from build123d import *
from build123d.topology import SkipClean

# Parameters (mm, degrees)
SKETCH1_W              = 39.5
SKETCH1_H              = 29
BOSS_EXTRUDE1_DEPTH    = 2
SKETCH2_R              = 13.5
SKETCH2_R_2            = 8.5
BOSS_EXTRUDE2_DEPTH    = 10
SKETCH3_R              = 12.5
CUT_EXTRUDE1_DEPTH     = 2
SKETCH4_R              = 7.5
CUT_EXTRUDE2_DEPTH     = 9
CUT_EXTRUDE3_START     = -10.3
CUT_EXTRUDE3_DEPTH     = 20.6
BOSS_EXTRUDE3_DEPTH    = 10
SKETCH10_W             = 39.5
SKETCH10_H             = 29
SKETCH10_R             = 13.5
CUT_EXTRUDE4_DEPTH     = 10
SKETCH11_R             = 13.5
SKETCH11_W             = 14
SKETCH11_H             = 20.6
BOSS_EXTRUDE4_DEPTH    = 8
SKETCH12_R             = 13.5
SKETCH12_R_2           = 12.5
BOSS_EXTRUDE5_DEPTH    = 2
CUT_SWEEP2_START       = -214.83981443
CUT_SWEEP2_OUTLINE_R   = 0.6
CUT_SWEEP2_DEPTH       = 22.83981443
CUT_SWEEP2_2_OUTLINE_R = 0.6
CUT_SWEEP2_2_ANGLE     = 17.195102
CUT_SWEEP2_START_2     = -205
CUT_SWEEP2_3_OUTLINE_R = 0.6
CUT_SWEEP2_3_DEPTH     = 2.526605635
BOSS_EXTRUDE7_DEPTH    = 10.25
CUT_EXTRUDE5_DEPTH     = 8
SKETCH20_R             = 1.6
CUT_EXTRUDE6_DEPTH     = 4
SKETCH21_R             = 2.5
SKETCH21_R_2           = 1.6
BOSS_EXTRUDE8_DEPTH    = 4
SKETCH22_W             = 4
SKETCH22_H             = 4
BOSS_EXTRUDE9_DEPTH    = 27
BOSS_EXTRUDE11_DEPTH   = 10
SKETCH8_2_R            = 0.6
SKETCH24_R             = 1.1
CUT_EXTRUDE7_DEPTH     = 1.1


with BuildPart() as part:
    # Sketch1 → Boss-Extrude1 (new body)
    with BuildSketch(Plane(origin=(0, 0, 0), x_dir=(1, 0, 0), z_dir=(0, 1, 0))):
        with Locations((-212.126239175, -24.349172792)):
            Rectangle(SKETCH1_W, SKETCH1_H)
    extrude(amount=BOSS_EXTRUDE1_DEPTH)

    # Sketch2 → Boss-Extrude2 (add)
    with BuildSketch(Plane(origin=(0, 2, 0), x_dir=(1, 0, 0), z_dir=(0, 1, 0))):
        with Locations((-206.876239175, -24.349172792)):
            Circle(SKETCH2_R)
        with Locations((-222.376239175, -24.349172792)):
            Circle(SKETCH2_R_2)
    extrude(amount=BOSS_EXTRUDE2_DEPTH)

    # Sketch3 → Cut-Extrude1 (cut)
    with BuildSketch(Plane(origin=(0, 12, 0), x_dir=(1, 0, 0), z_dir=(0, 1, 0))):
        with Locations(Location((-206.876239175, -24.349172792, 0), (0, 0, 270))):
            Circle(SKETCH3_R)
    extrude(amount=-CUT_EXTRUDE1_DEPTH, mode=Mode.SUBTRACT)

    # Sketch4 → Cut-Extrude2 (cut)
    with BuildSketch(Plane(origin=(0, 12, 0), x_dir=(1, 0, 0), z_dir=(0, 1, 0))):
        with Locations(Location((-222.376239175, -24.349172792, 0), (0, 0, 270))):
            Circle(SKETCH4_R)
    extrude(amount=-CUT_EXTRUDE2_DEPTH, mode=Mode.SUBTRACT)

    # Cut-Extrude3: read off the stored shape, not the designer's step
    # Cut-Extrude3 outline → Cut-Extrude3 (cut)
    with BuildSketch(Plane.XY.offset(24.349172792).offset(CUT_EXTRUDE3_START)):
        with BuildLine():
            ThreePointArc((-213.876239175, 8), (-206.876239175, 1), (-199.876239175, 8))
            Line((-199.876239175, 8), (-199.876239175, 10))
            Line((-199.876239175, 10), (-213.876239175, 10))
            Line((-213.876239175, 10), (-213.876239175, 8))
        make_face()
    extrude(amount=CUT_EXTRUDE3_DEPTH, mode=Mode.SUBTRACT)

    # Sketch7 → Boss-Extrude3 (add)
    with BuildSketch(Plane(origin=(0, 2, 0), x_dir=(1, 0, 0), z_dir=(0, 1, 0))):
        with BuildLine():
            Line((-192.376239175, -26.349172792), (-192.376239175, -24.349172792))
            Line((-192.376239175, -24.349172792), (-192.376239175, -22.349172792))
            Line((-192.376239175, -22.349172792), (-193.525209252, -22.349172792))
            ThreePointArc((-193.525209252, -22.349172792), (-193.413533207, -23.346402619), (-193.376239175, -24.349172792))
            ThreePointArc((-193.376239175, -24.349172792), (-193.413533207, -25.351942966), (-193.525209252, -26.349172792))
            Line((-193.525209252, -26.349172792), (-192.376239175, -26.349172792))
        make_face()
    extrude(amount=BOSS_EXTRUDE3_DEPTH)

    # Sketch10 → Cut-Extrude4 (cut)
    with BuildSketch(Plane(origin=(0, 2, 0), x_dir=(1, 0, 0), z_dir=(0, 1, 0))):
        with Locations((-212.126239175, -24.349172792)):
            Rectangle(SKETCH10_W, SKETCH10_H)
        with Locations(Location((-206.876239175, -24.349172792, 0), (0, 0, 151.062655238))):
            Circle(SKETCH10_R, mode=Mode.SUBTRACT)
    extrude(amount=CUT_EXTRUDE4_DEPTH, mode=Mode.SUBTRACT)

    # Sketch11 → Boss-Extrude4 (add)
    with BuildSketch(Plane(origin=(0, 2, 0), x_dir=(1, 0, 0), z_dir=(0, 1, 0))):
        with Locations(Location((-206.876239175, -24.349172792, 0), (0, 0, 151.062655238))):
            Circle(SKETCH11_R)
        with Locations((-206.876239175, -24.349172792)):
            Rectangle(SKETCH11_W, SKETCH11_H, mode=Mode.SUBTRACT)
    extrude(amount=BOSS_EXTRUDE4_DEPTH)

    # Sketch12 → Boss-Extrude5 (add)
    with SkipClean():  # the faces are left unmerged after this step: merging them gives an invalid solid
        with BuildSketch(Plane(origin=(0, 10, 0), x_dir=(1, 0, 0), z_dir=(0, 1, 0))):
            with Locations(Location((-206.876239175, -24.349172792, 0), (0, 0, 270))):
                Circle(SKETCH12_R)
            with Locations(Location((-206.876239175, -24.349172792, 0), (0, 0, 270))):
                Circle(SKETCH12_R_2, mode=Mode.SUBTRACT)
        extrude(amount=BOSS_EXTRUDE5_DEPTH)
    add(part.part.scale(1), mode=Mode.REPLACE)  # the faces are merged on a copy

    # Cut-Sweep2: read off the stored shape, not the designer's step
    # Cut-Sweep2 outline → Cut-Sweep2 (cut)
    with SkipClean():  # the faces are left unmerged after this step: merging them gives an invalid solid
        with BuildSketch(Plane.YZ.offset(CUT_SWEEP2_START)):
            with Locations((8.75, 24.349172792)):
                Circle(CUT_SWEEP2_OUTLINE_R)
        extrude(amount=CUT_SWEEP2_DEPTH, mode=Mode.SUBTRACT)

    # Cut-Sweep2 2 outline → Cut-Sweep2 2 (revolve, cut)
    with SkipClean():  # the faces are left unmerged after this step: merging them gives an invalid solid
        with BuildSketch(Plane(origin=(-214.83981433, 0, 9.349172792), x_dir=(-0.2956263792524328, 0, 0.9553036396298806), z_dir=(-0.9553036396298806, 0, -0.2956263792524328))):
            with Locations((15, 8.75)):
                Circle(CUT_SWEEP2_2_OUTLINE_R)
        revolve(axis=Axis((-214.83981433, 0, 9.349172792), (0, 1, 0)), revolution_arc=CUT_SWEEP2_2_ANGLE, mode=Mode.SUBTRACT)

    # Cut-Sweep2 3 outline → Cut-Sweep2 3 (cut)
    with SkipClean():  # the faces are left unmerged after this step: merging them gives an invalid solid
        with BuildSketch(Plane(origin=(0, 0, 0), x_dir=(0, 1, 0), z_dir=(0.9553036396298961, 0, 0.29562637925238305)).offset(CUT_SWEEP2_START_2)):
            with Locations((8.75, 87.443615225)):
                Circle(CUT_SWEEP2_3_OUTLINE_R)
        extrude(amount=CUT_SWEEP2_3_DEPTH, mode=Mode.SUBTRACT)

    # Sketch18 → Boss-Extrude7 (add)
    with SkipClean():  # the faces are left unmerged after this step: merging them gives an invalid solid
        with BuildSketch(Plane(origin=(0, 2, 0), x_dir=(1, 0, 0), z_dir=(0, 1, 0))):
            Polygon((-228.567210955, -11.746276031), (-229.459691419, -19.696337579), (-226.478418338, -20.031017753), (-225.585937874, -12.080956204), align=None)
            Polygon((-225.585937874, -12.080956204), (-226.478418338, -20.031017753), (-223.497145257, -20.365697927), (-222.604664794, -12.415636378), align=None)
            Polygon((-227.482458859, -28.974836995), (-226.92465857, -24.006048527), (-229.90593165, -23.671368353), (-230.46373194, -28.640156821), align=None)
            Polygon((-223.943385489, -24.340728701), (-226.92465857, -24.006048527), (-227.482458859, -28.974836995), (-224.501185779, -29.309517169), align=None)
        extrude(amount=BOSS_EXTRUDE7_DEPTH)

    # Sketch19 → Cut-Extrude5 (cut)
    with SkipClean():  # the faces are left unmerged after this step: merging them gives an invalid solid
        with BuildSketch(Plane(origin=(-5.039382401, 0, 44.889946486), x_dir=(0.9937576935397466, 0, 0.11156005795338761), z_dir=(-0.11156005795338761, 0, 0.9937576935397466))):
            Polygon((-222.830009143, 12.25), (-224.430009143, 12.25), (-224.430009143, 10.65), (-221.230009143, 10.65), (-221.230009143, 12.25), align=None)
        extrude(amount=-CUT_EXTRUDE5_DEPTH, mode=Mode.SUBTRACT)

    # Sketch20 → Cut-Extrude6 (cut)
    with SkipClean():  # the faces are left unmerged after this step: merging them gives an invalid solid
        with BuildSketch(Plane(origin=(-5.485622633, 0, 48.864977261), x_dir=(-0.9937576935397466, 0, -0.11156005795338761), z_dir=(0.11156005795338761, 0, -0.9937576935397466))):
            with Locations((222.830009143, 12.25)):
                Circle(SKETCH20_R)
        extrude(amount=-CUT_EXTRUDE6_DEPTH, mode=Mode.SUBTRACT)

    # Sketch21 → Boss-Extrude8 (add)
    with SkipClean():  # the faces are left unmerged after this step: merging them gives an invalid solid
        with BuildSketch(Plane(origin=(-5.485622633, 0, 48.864977261), x_dir=(-0.9937576935397466, 0, -0.11156005795338761), z_dir=(0.11156005795338761, 0, -0.9937576935397466))):
            with Locations((222.830009143, 12.25)):
                Circle(SKETCH21_R)
            with Locations((222.830009143, 12.25)):
                Circle(SKETCH21_R_2, mode=Mode.SUBTRACT)
        extrude(amount=-BOSS_EXTRUDE8_DEPTH)

    # Sketch22 → Boss-Extrude9 (add)
    with SkipClean():  # the faces are left unmerged after this step: merging them gives an invalid solid
        with BuildSketch(Plane(origin=(0, 2, 0), x_dir=(1, 0, 0), z_dir=(0, 1, 0))):
            with Locations((-229.876239175, -11.849172792)):
                Rectangle(SKETCH22_W, SKETCH22_H)
            with Locations((-229.876239175, -36.849172792)):
                Rectangle(SKETCH22_W, SKETCH22_H)
            with Locations((-194.376239175, -36.849172792)):
                Rectangle(SKETCH22_W, SKETCH22_H)
            with Locations((-194.376239175, -11.849172792)):
                Rectangle(SKETCH22_W, SKETCH22_H)
        extrude(amount=BOSS_EXTRUDE9_DEPTH)

    # Sketch23 → Boss-Extrude11 (add)
    with BuildSketch(Plane(origin=(0, 2, 0), x_dir=(1, 0, 0), z_dir=(0, 1, 0))):
        with BuildLine():
            Line((-193.376239175, -24.349172792), (-192.376239175, -24.349172792))
            Line((-192.376239175, -24.349172792), (-192.376239175, -22.349172792))
            Line((-192.376239175, -22.349172792), (-193.525209252, -22.349172792))
            ThreePointArc((-193.525209252, -22.349172792), (-193.413533207, -23.346402619), (-193.376239175, -24.349172792))
        make_face()
        with BuildLine():
            Line((-192.376239175, -26.349172792), (-192.376239175, -24.349172792))
            Line((-192.376239175, -24.349172792), (-193.376239175, -24.349172792))
            ThreePointArc((-193.376239175, -24.349172792), (-193.413533207, -25.351942966), (-193.525209252, -26.349172792))
            Line((-193.525209252, -26.349172792), (-192.376239175, -26.349172792))
        make_face()
    extrude(amount=BOSS_EXTRUDE11_DEPTH)

    # Cut-Sweep3: sweep along a path in Sketch17<2>
    with SkipClean():  # the faces are left unmerged after this step: merging them gives an invalid solid
        with BuildLine(Plane(origin=(0, 8.75, 0), x_dir=(1, 0, 0), z_dir=(0, 1, 0))) as cut_sweep3_path:
            Line((-192.376239175, -24.349172792), (-213.876239175, -24.349172792))
            Line((-213.876239175, -24.349172792), (-214.83981433, -24.349172792))
            ThreePointArc((-214.83981433, -24.349172792), (-217.08221049, -24.180614376), (-219.274210018, -23.678727387))
            Line((-219.274210018, -23.678727387), (-220.339151193, -23.349172792))
        # Sketch8<2> → Cut-Sweep3 (sweep, cut)
        with BuildSketch(Plane(origin=(-192.376239175, 0, 0), x_dir=(0, 0, -1), z_dir=(1, 0, 0))):
            with Locations((-24.349172792, 8.75)):
                Circle(SKETCH8_2_R)
        sweep(path=cut_sweep3_path.line, mode=Mode.SUBTRACT)
    add(part.part.scale(1), mode=Mode.REPLACE)  # the faces are merged on a copy

    # Sketch24 → Cut-Extrude7 (cut)
    with BuildSketch(Plane(origin=(0, 29, 0), x_dir=(1, 0, 0), z_dir=(0, 1, 0))):
        with Locations(Location((-229.876239175, -11.849172792, 0), (0, 0, 270))):
            Circle(SKETCH24_R)
        with Locations(Location((-229.876239175, -36.849172792, 0), (0, 0, 270))):
            Circle(SKETCH24_R)
        with Locations(Location((-194.376239175, -36.849172792, 0), (0, 0, 270))):
            Circle(SKETCH24_R)
        with Locations(Location((-194.376239175, -11.849172792, 0), (0, 0, 270))):
            Circle(SKETCH24_R)
    extrude(amount=-CUT_EXTRUDE7_DEPTH, mode=Mode.SUBTRACT)


solid = part.part
Build history of the part. All positions in model axes, mm. A direction names the side the tool comes from. Round coordinates to 2 decimals unless told otherwise and drop trailing zeros. Write each loop counter-clockwise with the first axis right and the second up, starting at its lowest first coordinate (ties: lowest second). Pieces come first, ordered by that corner, then holes. Notation, with made-up numbers: M -35,15.25 L -26,15.25 A20 ccw -26,30.25 Z; hole C 25.25,84 d6. An arc over 180 degrees is marked long. Answer as a JSON object with one key per item and string values. Group by question number.
(1) Cut at A-A (y = 19.5). Give the cut face in (x, z).
(2) Flat gauge pins, fed straight in: pin 1 (2.5 mm diameter, centred on x = -194.5, z = 37, fed in from +Y); pin 2 (0.7 mm diameter, centred on x = -223.5, z = 15.5, fed in from +Y); pin 3 (3 mm diameter, centred on y = 9.5, z = 19, fed in from +X); pin 4 (1 mm diameter, centred on y = 8.5, z = 20, fed in from -X). Where does each tip first touch, or does it go through?
(3) Cut at B-B (x = -208.5). Give the cut face in (y, z).
(4) Which spindle directions (+Z, -Z, +X, -X, +Y, -Y) get a long thin tool onto all of the face, cutting with end or side? Do faces 1 (the flat face through (-224.45, 11.44, 16.29)), 2 (the flat face through (-230, 15, 34.849)), 3 (the flat face through (-194, 15, 13.849)), 4 (the flat face through (-207, 7, 14.049)), 5 (the flat face through (-224.226, 7.053, 26.86)). Say none if no direction does.
(5) Cut at C-C (z = 19). Give the cut face in (x, y).
(6) Cut at D-D (y = 2.5). Give the number of separate pieces and of enclosed holes in the cut face, and give its area (3 significant figures).
(7) Mould opens along X. For faces 6 (the flat face through (-212, 0, 24)), 7 (the flat face through (-196.376, 15, 37)), 8 (the flat face through (-230.18, 7.05, 26.12)) say: pulls with the +X half, pulls with the -X half, needs draft (parallel to the pull), parting line crosses it, or undercut.
(8) Drill centre lines: L1, parallel to Z at x = -192.65, y = 8.75; L2, parallel to Z at x = -207, y = 11.5; L3, parallel to Z at x = -229, y = 24. Where is each one in solid material? Low to high.
Responses:
{
 "1": {"outline": "M -231.88,9.85 L -227.88,9.85 L -227.88,13.85 L -231.88,13.85 Z; M -231.88,34.85 L -227.88,34.85 L -227.88,38.85 L -231.88,38.85 Z; M -196.38,9.85 L -192.38,9.85 L -192.38,13.85 L -196.38,13.85 Z; M -196.38,34.85 L -192.38,34.85 L -192.38,38.85 L -196.38,38.85 Z"},
 "2": {"pin 1": "stops at y = 29", "pin 2": "stops at y = 12.25", "pin 3": "stops at x = -193.94", "pin 4": "stops at x = -229.46"},
 "3": {"outline": "M 0,9.85 L 2,9.85 L 2,10.95 L 12,10.95 L 12,11.96 L 10,11.96 L 10,14.05 L 1.19,14.05 L 1.19,34.65 L 10,34.65 L 10,36.74 L 12,36.74 L 12,37.75 L 2,37.75 L 2,38.85 L 0,38.85 Z"},
 "4": {"face 1": "-Z, +Y", "face 2": "-X, +Y", "face 3": "+X, +Y", "face 4": "+Y", "face 5": "+Z, +Y"},
 "5": {"outline": "M -231.88,0 L -192.38,0 L -192.38,2 L -194.48,2 L -194.48,12 L -195.58,12 L -195.58,10 L -199.88,10 L -199.88,8 A7 cw -213.88,8 L -213.88,10 L -218.17,10 L -218.17,12 L -219.27,12 L -219.27,2 L -223.34,2 L -223.34,12.25 L -224.75,12.25 L -224.75,10.65 L -227.97,10.65 L -227.97,12.25 L -229.38,12.25 L -229.38,2 L -231.88,2 Z"},
 "6": {"separate pieces": "6", "enclosed holes": "1", "area": "539 mm2"},
 "7": {"face 6": "needs draft", "face 7": "undercut", "face 8": "pulls with the -X half"},
 "8": {"L1": "z = 9.85 to 13.85, 22.35 to 23.75, 24.95 to 26.35, 34.85 to 38.85", "L2": "z = 10.85 to 11.85, 36.85 to 37.85", "L3": "z = 9.85 to 13.85, 34.85 to 38.85"}
}
